Check sheet for the modelled part. Datum: model origin and axes. Units: mm. Face numbers are marked on the shaded views. A direction names the side the tool comes from. Round coordinates to 2 decimals unless told otherwise and drop trailing zeros. Loops run counter-clockwise (first coordinate to the right, second up) from the corner with the lowest first, then second, coordinate; pieces in that order, holes last. Notation, with made-up numbers: (44, -3) - (96, -3) arc R17 cw to (96, 6) - close; hole circle Ø7 at (1, 74). An arc over 180 degrees is marked (long way). Put each result on its own line as item: value.
Autodesk Inventor part; units mm, degrees
ref_plane "YZ Plane" through (0, 0, 0) normal (1, 0, 0) x (0, 1, 0)
ref_plane "XZ Plane" through (0, 0, 0) normal (0, 1, 0) x (-1, 0, 0)
ref_plane "XY Plane" through (0, 0, 0) normal (0, 0, 1) x (1, 0, 0)
sketch "Sketch1" plane through (0, 0, 0) normal (0, 1, 0) x (-1, 0, 0)
  line L0 (-23, 55) -> (23, 55)
  line L1 (23, 55) -> (23, -55)
  line L2 (23, -55) -> (-23, -55)
  line L3 (-23, -55) -> (-23, 55)
  line L4 (-23, 55) -> (23, -55) construction
  line L5 (23, 55) -> (-23, -55) construction
  point P0 (0, 0)
  dimension "d0" = 46
  dimension "d1" = 110
extrude "Extrusion1" add sketch "Sketch1" along normal blind 3
sketch "Sketch2" plane through (0, 3, 0) normal (0, 1, 0) x (1, 0, 0)
  line L0 (-23, 55) -> (-23, -55)
  line L1 (23, -55) -> (-23, -55)
  line L2 (-23, -55) -> (-23, 55)
  line L3 (-23, 55) -> (23, 55)
  line L4 (23, 55) -> (23, -55)
  line L5 (23, -55) -> (-23, 55) construction
  line L6 (-23, -55) -> (23, 55) construction
  line L7 (21, -53) -> (-21, -53)
  line L8 (-21, -53) -> (-21, 53)
  line L9 (-21, 53) -> (21, 53)
  line L10 (21, 53) -> (21, -53)
  line L11 (21, -53) -> (-21, 53) construction
  line L12 (-21, -53) -> (21, 53) construction
  point P0 (0, 0)
  dimension "d4" = 42
  dimension "d5" = 106
extrude "Extrusion2" add sketch "Sketch2" along normal blind 30
sketch "Sketch5" plane through (0, 33, 0) normal (0, 1, 0) x (1, 0, 0)
  line L0 (23, 55) -> (-23, 55)
  line L1 (23, -55) -> (23, 55)
  line L2 (-23, 55) -> (-23, -55)
  line L3 (21, 53) -> (21, -53)
  line L4 (21, -42) -> (23, -42)
  line L5 (23, -42) -> (23, -3)
  line L6 (23, -3) -> (21, -3)
  line L7 (21, -3) -> (21, -42)
  line L8 (-23, -55) -> (23, -55)
  point P0 (0, 0)
  point P1 (22, -42)
  point P2 (22, -3)
  dimension "d24" = 13
  dimension "d25" = 58
extrude "Extrusion5" cut sketch "Sketch5" against normal blind 18 contours L1 L4 L3 L6
sketch "Sketch6" plane through (23, 0, -55) normal (0, 0, -1) x (-1, 0, 0)
  line L0 (15, 22) -> (31, 22)
  line L1 (31, 22) -> (31, 12)
  line L2 (31, 12) -> (15, 12)
  line L3 (15, 12) -> (15, 22)
  line L4 (46, 0) -> (46, 33)
  line L5 (0, 0) -> (46, 0)
  point P0 (23, 0)
  dimension "d28" = 16
  dimension "d29" = 15
  dimension "d30" = 10
  dimension "d32" = 12
extrude "Extrusion6" cut sketch "Sketch6" against normal blind 15
sketch "Sketch7" plane through (-23, 0, 55) normal (0, 0, 1) x (1, 0, 0)
  line L0 (5, 25) -> (31, 25)
  line L1 (31, 25) -> (31, 15)
  line L2 (31, 15) -> (5, 15)
  line L3 (5, 15) -> (5, 25)
  line L4 (0, 0) -> (0, 33)
  line L5 (0, 0) -> (46, 0)
  point P0 (23, 0)
  dimension "d35" = 5
  dimension "d36" = 10
  dimension "d37" = 15
  dimension "d38" = 26
extrude "Extrusion7" cut sketch "Sketch7" against normal blind 15
sketch "Sketch9" plane through (0, 33, 0) normal (0, 1, 0) x (1, 0, 0)
  circle A0 centre (0, -60) radius 2
  line L0 (-23, -55) -> (23, -55)
  line L1 (4, -55) -> (-4, -55)
  line L2 (-4, -55) -> (-4, -60)
  line L3 (4, -60) -> (4, -55)
  arc A1 (-4, -60) -> (4, -60) centre (0, -60) ccw
  circle A2 centre (0, 60) radius 2
  line L4 (23, 55) -> (-23, 55)
  line L5 (4, 55) -> (-4, 55)
  line L6 (-4, 55) -> (-4, 60)
  line L7 (4, 60) -> (4, 55)
  arc A3 (4, 60) -> (-4, 60) centre (0, 60) ccw
  point P0 (0, 0)
  point P1 (0, -55)
  point P2 (0, -55)
  point P3 (0, 55)
  point P4 (0, 55)
  point P5 (0, 55)
  dimension "d77" = 4
  dimension "d78" = 5
  dimension "d79" = 8
  dimension "d80" = 4
  dimension "d81" = 4
  dimension "d82" = 4
  dimension "d83" = 5
  dimension "d84" = 8
  dimension "d85" = 4
extrude "Extrusion10" [suppressed]
fillet "Fillet2" [suppressed]
sketch "Sketch11" plane through (0, 3, 0) normal (0, 1, 0) x (1, 0, 0)
  circle A0 centre (-17.5, 47.75) radius 1
  circle A1 centre (17.5, 47.75) radius 1
  circle A2 centre (-17.5, -47.75) radius 1
  circle A3 centre (17.5, -47.75) radius 1
  line L0 (-21, 53) -> (-21, -53)
  line L1 (-21, 53) -> (-15, 53)
  line L2 (-15, 53) -> (-15, 46)
  line L3 (-15, 46) -> (-21, 46)
  line L4 (-21, 46) -> (-21, 53)
  line L5 (21, 53) -> (-21, 53)
  line L6 (21, 53) -> (15, 53)
  line L7 (15, 53) -> (15, 46)
  line L8 (15, 46) -> (21, 46)
  line L9 (21, 46) -> (21, 53)
  line L10 (-21, -53) -> (-15, -53)
  line L11 (-15, -53) -> (-15, -46)
  line L12 (-15, -46) -> (-21, -46)
  line L13 (-21, -46) -> (-21, -53)
  line L14 (21, -53) -> (15, -53)
  line L15 (15, -53) -> (15, -46)
  line L16 (15, -46) -> (21, -46)
  line L17 (21, -46) -> (21, -53)
  point P0 (0, 0)
  dimension "d95" = 2
  dimension "d96" = 2
  dimension "d97" = 2
  dimension "d98" = 2
  dimension "d99" = 95.5
  dimension "d100" = 35
  dimension "d101" = 47.75
  dimension "d102" = 17.5
  dimension "d103" = 6
  dimension "d104" = 7
  dimension "d105" = 6
  dimension "d106" = 7
  dimension "d107" = 6
  dimension "d108" = 7
  dimension "d109" = 6
  dimension "d110" = 7
extrude "Extrusion11" add sketch "Sketch11" along normal blind 11
fillet "Fillet6" radius 2 20 edges at (-23, 16.5, -55) (-23, 16.5, 55) (23, 16.5, 55) (23, 16.5, -55) (21, 23.5, -53) (-21, 23.5, -53) (-21, 23.5, 53) (21, 23.5, 53) (15, 8.5, -46) (-15, 8.5, -46) (15, 8.5, 46) (-15, 8.5, 46) (21, 8.5, -46) (15, 8.5, -53) (-15, 8.5, -53) (-21, 8.5, -46) (-21, 8.5, 46) (-15, 8.5, 53) (21, 8.5, 46) (15, 8.5, 53)
sketch "Sketch12" plane through (0, 0, 0) normal (0, -1, 0) x (1, 0, 0)
  line L0 (0, 50) -> (0, 60) construction
  line L1 (-21, 55) -> (21, 55)
  line L2 (4, 50) -> (4, 60)
  line L3 (-4, 60) -> (-4, 50)
  arc A0 (-4, 50) -> (4, 50) centre (0, 50) ccw
  arc A1 (4, 60) -> (-4, 60) centre (0, 60) ccw
  circle A2 centre (0, 60) radius 2
  point P0 (0, 0)
  point P1 (0, 55)
  point P2 (-4, 55)
  point P3 (4, 55)
  dimension "d115" = 5
  dimension "d116" = 8
  dimension "d117" = 4
extrude "Extrusion12" add sketch "Sketch12" against normal blind 6 contours L3 A1 L2 L1
mirror "Mirror1" about plane through (0, 0, 0) normal (0, 0, 1) of "Extrusion12"
properties part number "M12StereoPiBracket"
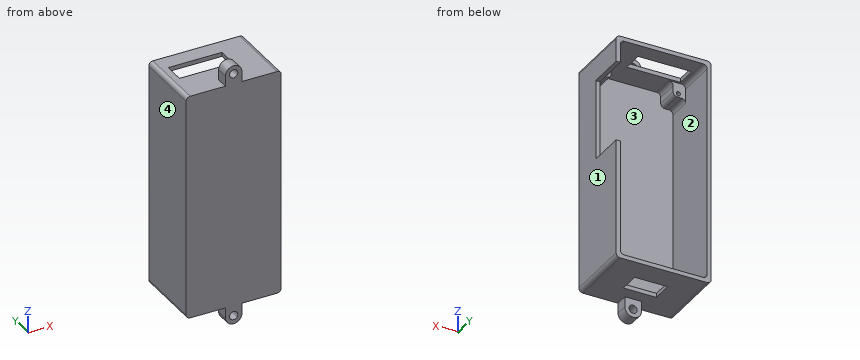
Item 1: Thickness scan on line 1 (X direction, y = 8.5, z = -47.75); line 2 (Z direction, x = 3, y = 6.5); line 3 (X direction, y = 9, z = -39.5). Record the ranges inside material, lowest first. Write a range as from..to.
Filled sheet:
line 1: -23..-18.5, -16.5..-15.02, 15.02..16.5, 18.5..23
line 2: -55..-53, 53..55
line 3: -23..-21, 21..23
Item 2: Go/stop test with flat-tipped pins: pin 1 (4 mm diameter, centred on x = -1.5, z = 59, fed in from +Y); pin 2 (3 mm diameter, centred on x = -13.5, y = 29.5, fed in from +Z); pin 3 (4 mm diameter, centred on y = 4, z = -57.5, fed in from -X). Record where each tip stops, or that it passes through.
Filled sheet:
pin 1: y = 6
pin 2: z = 55
pin 3: x = -4
Item 3: Section check D-D on y = 30.5. Enter the section's corners in (x, z), then the cut area to 3 significant figures.
Filled sheet:
outline: (-23, -53) arc R2 ccw to (-21, -55) - (21, -55) arc R2 ccw to (23, -53) - (23, 3) - (21, 3) - (21, -51) arc R2 cw to (19, -53) - (-19, -53) arc R2 cw to (-21, -51) - (-21, 51) arc R2 cw to (-19, 53) - (19, 53) arc R2 cw to (21, 51) - (21, 42) - (23, 42) - (23, 53) arc R2 ccw to (21, 55) - (-21, 55) arc R2 ccw to (-23, 53) - close
area: 530 mm²
Item 4: Release check for a two-part mould opening along Z. For the marked faces 1 and 2 record: +Z half, -Z half, draft (parallel to the pull), parting line (faces both ways), or undercut.
Filled sheet:
face 1: draft
face 2: undercut
Item 5: Tool access check on the marked faces 3 and 4. Record the directions out of +Z, -Z, +X, -X, +Y, -Y that give a thin tool (end or side, any length) a straight path to the whole face; none if there is none.
Filled sheet:
face 3: +Y
face 4: +Z, -Z, -X, +Y, -Y
Item 6: Section check B-B on y = 20. Enter the section's corners in (x, z).
Filled sheet:
outline: (-23, -53) arc R2 ccw to (-21, -55) - (-8, -55) - (-8, -53) - (-19, -53) arc R2 cw to (-21, -51) - (-21, 51) arc R2 cw to (-19, 53) - (-18, 53) - (-18, 55) - (-21, 55) arc R2 ccw to (-23, 53) - close; (8, -55) - (21, -55) arc R2 ccw to (23, -53) - (23, 3) - (21, 3) - (21, -51) arc R2 cw to (19, -53) - (8, -53) - close; (8, 53) - (19, 53) arc R2 cw to (21, 51) - (21, 42) - (23, 42) - (23, 53) arc R2 ccw to (21, 55) - (8, 55) - close
Item 7: Section check A-A on x = 0. Enter the section's corners in (y, z).
Filled sheet:
outline: (0, -64) - (6, -64) - (6, -62) - (0, -62) - close; (0, -58) - (6, -58) - (6, -55) - (12, -55) - (12, -53) - (3, -53) - (3, 53) - (15, 53) - (15, 55) - (6, 55) - (6, 58) - (0, 58) - close; (0, 62) - (6, 62) - (6, 64) - (0, 64) - close; (22, -55) - (33, -55) - (33, -53) - (22, -53) - close; (25, 53) - (33, 53) - (33, 55) - (25, 55) - close
Item 8: Section check C-C on z = -37.5. Enter the section's corners in (x, y).
Filled sheet:
outline: (-23, 0) - (23, 0) - (23, 33) - (21, 33) - (21, 3) - (-21, 3) - (-21, 33) - (-23, 33) - close
